Geometry check sheet. Reference: the model listing, model coordinates, mm. Face numbers are marked on the shaded views. A direction names the side the tool comes from. Round coordinates to 2 decimals unless told otherwise and drop trailing zeros. Write each loop counter-clockwise with the first axis right and the second up, starting at its lowest first coordinate (ties: lowest second). Pieces come first, ordered by that corner, then holes. Notation, with made-up numbers: (69, 81.5) -> (122, 81.5) arc R30 cw to (122, 117.5) -> close; hole circle Ø4 at (70, 64.25). An arc over 180 degrees is marked (long way). Return JSON: item names as keys, results as strings. Group by question number.
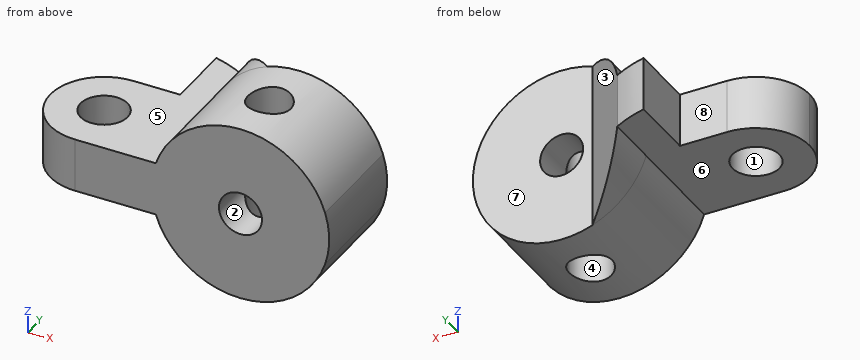
from build123d import *
from build123d.topology import SkipClean

# Parameters (mm, degrees)
SKETCH1_R               = 1.6
BOSS_EXTRUDE1_DEPTH     = 8
CUT_EXTRUDE1_DEPTH      = 21.082666196
CUT_EXTRUDE1_DEPTH_BACK = 21.082666196
SKETCH2_R               = 1.75
SKETCH2_R_2             = 1.6
SKETCH4_W               = 2.5
SKETCH4_H               = 4
BOSS_EXTRUDE3_DEPTH     = 5
CHAMFER1_START          = 8
CHAMFER1_DEPTH          = 4
CHAMFER1_START_2        = -8
CHAMFER1_2_DEPTH        = 16
FILLET2_R               = 10


with BuildPart() as part:
    # Sketch1 → Boss-Extrude1 (new body)
    with BuildSketch(Plane(origin=(0, 0, 0), x_dir=(1, 0, 0), z_dir=(0, 1, 0))):
        with BuildLine():
            Line((-6.289674077, 2), (-16.289674077, 2))
            Line((-16.289674077, 2), (-16.289674077, -2))
            Line((-16.289674077, -2), (-6.289674077, -2))
            ThreePointArc((-6.289674077, -2), (0, -6.6), (6.289674077, -2))
            ThreePointArc((6.289674077, -2), (6.6, 0), (6.289674077, 2))
            ThreePointArc((6.289674077, 2), (0, 6.6), (-6.289674077, 2))
        make_face()
        with Locations(Location((0, 0, 0), (0, 0, 270))):
            Circle(SKETCH1_R, mode=Mode.SUBTRACT)
    extrude(amount=BOSS_EXTRUDE1_DEPTH)

    # Sketch2 → Cut-Extrude1 (cut, two sides: drawn at the far end of the back side and taken through both)
    with BuildSketch(Plane.XY.offset(2).offset(-CUT_EXTRUDE1_DEPTH_BACK)):
        with BuildLine():
            Line((-16.289674077, 8), (-16.289674077, 4))
            ThreePointArc((-16.289674077, 4), (-15.118101202, 6.828427125), (-12.289674077, 8))
            Line((-12.289674077, 8), (-16.289674077, 8))
        make_face()
        with BuildLine():
            Line((-16.289674077, 4), (-16.289674077, 0))
            Line((-16.289674077, 0), (-12.289674077, 0))
            ThreePointArc((-12.289674077, 0), (-15.118101202, 1.171572875), (-16.289674077, 4))
        make_face()
        with Locations(Location((-12.289674077, 4, 0), (0, 0, 180))):
            Circle(SKETCH2_R)
        with Locations((0, 4)):
            Circle(SKETCH2_R_2)
    extrude(amount=CUT_EXTRUDE1_DEPTH + CUT_EXTRUDE1_DEPTH_BACK, mode=Mode.SUBTRACT)

    # Sketch4 → Boss-Extrude3 (add)
    with BuildSketch(Plane(origin=(0, 8, 0), x_dir=(1, 0, 0), z_dir=(0, 1, 0))):
        with Locations((-7.539674077, 0)):
            Rectangle(SKETCH4_W, SKETCH4_H)
    extrude(amount=BOSS_EXTRUDE3_DEPTH)

    # Chamfer1: read off the stored shape, not the designer's step
    # Chamfer1 outline → Chamfer1 (add)
    with SkipClean():  # the faces are left unmerged after this step: merging them gives an invalid solid
        with BuildSketch(Plane(origin=(0, 0, 0), x_dir=(1, 0, 0), z_dir=(0, 1, 0)).offset(CHAMFER1_START)):
            with BuildLine():
                ThreePointArc((-6.289674077, -2), (6.6, 0), (-6.289674077, 2))
                Line((-6.289674077, 2), (-6.289674077, -2))
            make_face()
        extrude(amount=CHAMFER1_DEPTH)

    # Chamfer1 2 outline → Chamfer1 2 (cut)
    with BuildSketch(Plane.XY.offset(CHAMFER1_START_2)):
        Polygon((-2.289674077, 8), (8, 8), (8, 12), (-6.289674077, 12), align=None)
    extrude(amount=CHAMFER1_2_DEPTH, mode=Mode.SUBTRACT)

    # Fillet2
    # the kernel refuses this fillet: 10 mm, written as the material it takes off along each edge
    with BuildSketch(Plane(origin=(-6.289674077, 13, -8.25), x_dir=(4.06555678011955e-10, -1.0, 0), z_dir=(0, 0, 1))) as fillet2_piece_1:
        with BuildLine():
            CenterArc((9.700238938, -4.930095579), FILLET2_R, 150.461416233, 15.474348521)
            Line((-1e-09, -2.5), (0, 0))
            Line((0, 0), (1, 0))
        make_face()
    extrude(amount=16.5, mode=Mode.SUBTRACT)


solid = part.part
1) Sectioned sample at B-B on z = 1.25. Enter the section's corners in (x, y), and give its area (3 significant figures).
2) Sectioned sample at A-A on x = 0. Enter the section's corners in (y, z), and give its area (3 significant figures).
3) Mould release check, pull along Y, two halves, no side actions. Record for the marked faces 1, 2, 3 and 4: +Y half, -Y half, draft (parallel to the pull), parting line (faces both ways), or undercut.
4) Sectioned sample at C-C on y = 6.75. Enter the section's corners in (x, z), and give its area (3 significant figures).
5) Material ranges on probe 1 along Y at (x, z) = (0, -2); probe 2 along X at (y, z) = (5.1, 0); probe 3 along Y at (x, z) = (3.75, -4), recorded low to high. Write a range as [from, to].
6) Tool access check on the marked faces 5, 6, 7 and 8. Record the directions out of +Z, -Z, +X, -X, +Y, -Y that give a thin tool (end or side, any length) a straight path to the whole face; none if there is none.
7) Sectioned sample at D-D on z = -0.25. Enter the section's corners in (x, y), and give its area (3 significant figures).
8) Go/stop test with flat-tipped pins: P1, Ø5, axis at x = -13, y = 4, coming from the +Z side; P2, Ø1.5, axis at y = 5, z = 4.5, coming from the +X side; P3, Ø2, axis at y = 7.5, z = 0, coming from the -X side. Record where each tip stops, or that it passes through.
Evaluation:
{
 "1": {"outline": "(-12.29, 0) -> (-1, 0) -> (-1, 2.75) arc R1.6 cw to (-1, 5.25) -> (-1, 8) -> (-2.29, 8) -> (-6.29, 12) arc R10 ccw to (-8.79, 13) -> (-8.79, 8) -> (-12.29, 8) arc R4 ccw to start; (1, 0) -> (6.48, 0) -> (6.48, 8) -> (1, 8) -> (1, 5.25) arc R1.6 cw to (1, 2.75) -> close; hole circle Ø3.5 at (-12.29, 4)", "area": "167 mm2"},
 "2": {"outline": "(0, -6.6) -> (2.4, -6.6) -> (2.4, -1.6) -> (0, -1.6) -> close; (0, 1.6) -> (2.4, 1.6) -> (2.4, 6.6) -> (0, 6.6) -> close; (5.6, -6.6) -> (8, -6.6) -> (8, -1.6) -> (5.6, -1.6) -> close; (5.6, 1.6) -> (8, 1.6) -> (8, 6.6) -> (5.6, 6.6) -> close", "area": "48.0 mm2"},
 "3": {"face 1": "undercut", "face 2": "draft", "face 3": "+Y half", "face 4": "undercut"},
 "4": {"outline": "(-15.19, -2) -> (-6.29, -2) arc R6.6 ccw (long way) to (-6.29, 2) -> (-15.19, 2) -> close; hole circle Ø3.2 at (0, 0)", "area": "164 mm2"},
 "5": {"probe 1": "y = [0, 2.4], [5.6, 8]", "probe 2": "x = [-16.14, -13.65], [-10.93, -1.6], [1.6, 6.6]", "probe 3": "y = [0, 8]"},
 "6": {"face 5": "+Z, -X, +Y, -Y", "face 6": "-Z, -X, +Y, -Y", "face 7": "+Z, -Z, +X, +Y", "face 8": "+Z, -Z, -X, +Y"},
 "7": {"outline": "(-12.29, 0) -> (-1.58, 0) -> (-1.58, 3.75) arc R1.6 cw to (-1.58, 4.25) -> (-1.58, 8) -> (-2.29, 8) -> (-6.29, 12) arc R10 ccw to (-8.79, 13) -> (-8.79, 8) -> (-12.29, 8) arc R4 ccw to start; (1.58, 0) -> (6.6, 0) -> (6.6, 8) -> (1.58, 8) -> (1.58, 4.25) arc R1.6 cw to (1.58, 3.75) -> close; hole circle Ø3.5 at (-12.29, 4)", "area": "161 mm2"},
 "8": {"P1": "stops at z = 2", "P2": "stops at x = 5.43", "P3": "stops at x = -15.41"}
}
